from build123d import *

# Parameters (mm, degrees)
BASPROSKE_W         = 8
BASPROSKE_H         = 12.75
TOOTHCUT_DEPTH      = 20.726251545
TEETHCUTS_COUNT     = 15
TEETHCUTS_ANGLE     = 336
BORSKE_R            = 3
BORE_DEPTH          = 50.0000508
SKETCH2_R           = 3.2
CUT_EXTRUDE1_DEPTH  = 20.701035813
BOSS_EXTRUDE1_DEPTH = 8


with BuildPart() as part:
    # BasProSke → Base-Revolve (revolve)
    with BuildSketch(Plane(origin=(0, 0, 0), x_dir=(1, 0, 0), z_dir=(0, 1, 0)), mode=Mode.PRIVATE) as base_revolve_sk:
        with Locations((4, 6.375)):
            Rectangle(BASPROSKE_W, BASPROSKE_H)
    revolve(base_revolve_sk.sketch.rotate(Axis((-10, 0, 0), (1, 0, 0)), 180), axis=Axis((-10, 0, 0), (1, 0, 0)))

    # TooCutSke → ToothCut (cut, through all)
    with BuildSketch(Plane(origin=(0, 0, 0), x_dir=(0, 0, -1), z_dir=(1, 0, 0))):
        with BuildLine():
            ThreePointArc((0.791546546, 9.340520867), (0, 9.374), (-0.791546546, 9.340520867))
            ThreePointArc((-0.791546546, 9.340520867), (-1.235070734, 11.110218102), (-2.344732916, 12.558386549))
            ThreePointArc((-2.344732916, 12.558386549), (0, 12.7754), (2.344732916, 12.558386549))
            ThreePointArc((2.344732916, 12.558386549), (1.235070734, 11.110218102), (0.791546546, 9.340520867))
        make_face()
    toothcut = extrude(amount=TOOTHCUT_DEPTH, mode=Mode.SUBTRACT)

    # TeethCuts: ToothCut ×15 about axis
    teethcuts_axis = Axis((-10, 0, 0), (1, 0, 0))
    for i in range(1, TEETHCUTS_COUNT):
        add(toothcut.rotate(teethcuts_axis, i * TEETHCUTS_ANGLE / (TEETHCUTS_COUNT - 1)), mode=Mode.SUBTRACT)

    # BorSke → Bore (cut, symmetric)
    with BuildSketch(Plane(origin=(0, 0, 0), x_dir=(0, 0, -1), z_dir=(1, 0, 0))):
        with Locations(Location((0, 0, 0), (0, 0, 180))):
            Circle(BORSKE_R)
    extrude(amount=BORE_DEPTH, both=True, mode=Mode.SUBTRACT)

    # Sketch2 → Cut-Extrude1 (cut, through all)
    with BuildSketch(Plane.ZY):
        Circle(SKETCH2_R)
    extrude(amount=-CUT_EXTRUDE1_DEPTH, mode=Mode.SUBTRACT)

    # Sketch3 → Boss-Extrude1 (add)
    with BuildSketch(Plane.ZY):
        with BuildLine():
            Line((2.4, 2.116601049), (2.4, -2.116601049))
            ThreePointArc((2.4, -2.116601049), (3.2, 0), (2.4, 2.116601049))
        make_face()
    extrude(amount=-BOSS_EXTRUDE1_DEPTH)


solid = part.part
Source: CAD feature listing. Evaluate the final solid. Frame: model axes, mm. A direction names the side the tool comes from. Give positions to 0.01 mm unless a question says otherwise; leave off trailing zeros. Write each loop counter-clockwise with the first axis right and the second up, starting at its lowest first coordinate (ties: lowest second). Pieces come first, ordered by that corner, then holes. Notation, with made-up numbers: M -15,-37.75 L 28,-37.75 A35 ccw 28,-5.75 Z; hole C 23.25,-5 d7. An arc over 180 degrees is marked long. Return JSON: item names as keys, results as strings. Group by question number.
1) Set-up query: faces 1 (the face through (3.944, -10.618, 3.524)), 2 (the face through (3.944, 4.614, 10.191)), 3 (the face through (3.94, 9.65, -5.65)), 4 (the face through (3.944, 8.313, -7.414)), 5 (the face through (3.944, 2.257, -10.957)). Return all of +Z, -Z, +X, -X, +Y, -Y with unobstructed straight access to the full face (end or side cutting, diameter ignored); none if empty.
2) Cut plane B-B, the plane y = 4. Output: boundary loops of the cut face in (x, z), plus the area to 3 significant figures.
3) Cut plane A-A, the plane z = 0. Output: boundary loops of the cut face in (x, y).
4) Pin query (flat end, axial travel): P1, Ø2, axis at x = 3.5, z = -5, coming from the -Y side; P2, Ø1, axis at x = 1.5, y = -10, coming from the -Z side; P3, Ø1.5, axis at x = 3.5, y = 5.5, coming from the +Z side. Return the tip coordinate at first contact, or that it passes through.
5) Material intervals for line 1 along Z through (x, y) = (1.75, -10.25); line 2 along Z through (x, y) = (7, 8.5); line 3 along Z through (x, y) = (6, -5.25), sorted ascending. Write a range as [from, to].
6) Cut plane C-C, the plane y = 7.75. Output: boundary loops of the cut face in (x, z), plus the area to 3 significant figures.
7) Pull-direction query (Z, two-part tool) for faces 6 (the face through (3.944, -2.395, -10.928)), 7 (the face through (3.94, -6.59, 8.98)), 8 (the face through (3.944, -9.723, -5.533)); classes: pulls with the +Z half, pulls with the -Z half, needs draft (parallel to the pull), parting line crosses it, or undercut.
Recorded:
{
 "1": {"face 1": "+X, -X, -Y", "face 2": "+Z, +X, -X", "face 3": "+X, -X, +Y", "face 4": "-Z, +X, -X", "face 5": "+X, -X"},
 "2": {"outline": "M 0,-9.39 L 8,-9.39 L 8,9.39 L 0,9.39 Z", "area": "150 mm²"},
 "3": {"outline": "M 0,-12.75 L 8,-12.75 L 8,-3.2 L 0,-3.2 Z; M 0,3.2 L 8,3.2 L 8,9.37 L 0,9.37 Z"},
 "4": {"P1": "stops at y = -11.78", "P2": "stops at z = -5.6", "P3": "stops at z = 11.21"},
 "5": {"line 1": "z = [-5.6, -3.27], [-1.23, 1.23], [3.27, 5.6]", "line 2": "z = [-7.49, -4.68], [-3.95, 3.95], [4.68, 7.49]", "line 3": "z = [-7.77, 7.77]"},
 "6": {"outline": "M 0,-7.13 L 8,-7.13 L 8,7.13 L 0,7.13 Z", "area": "114 mm²"},
 "7": {"face 6": "pulls with the -Z half", "face 7": "pulls with the +Z half", "face 8": "undercut"}
}
